```python
from build123d import *

# Parameters (mm, degrees)
F0_W     = 107
F0_H     = 248
F0_W_2   = 99
F0_H_2   = 240
F1_DEPTH = 65
F2_W     = 107
F2_H     = 248
F2_W_2   = 99
F2_H_2   = 240
F3_DEPTH = 4
F4_W     = 58.7
F4_H     = 31.5
F5_DEPTH = 25
F6_R     = 3


with BuildPart() as f1:
    # F0 (on Front) → F1 (new body)
    with BuildSketch(Plane.XZ):
        with Locations((49.5, 120)):
            Rectangle(F0_W, F0_H)
        with Locations((49.5, 120)):
            Rectangle(F0_W_2, F0_H_2, mode=Mode.SUBTRACT)
    extrude(amount=F1_DEPTH)

    # F2 (on face) → F3 (join)
    with BuildSketch(Plane.XZ.offset(65)):
        with Locations((49.5, 120)):
            Rectangle(F2_W, F2_H)
        with Locations((49.5, 120)):
            Rectangle(F2_W_2, F2_H_2, mode=Mode.SUBTRACT)
        with Locations((49.5, 120)):
            Rectangle(F2_W_2, F2_H_2)
    extrude(amount=F3_DEPTH)

    # F4 (on face) → F5 (cut)
    with BuildSketch(Plane.XZ.offset(69)):
        with Locations((49.35, 202.9458682446)):
            Rectangle(F4_W, F4_H)
    extrude(amount=-F5_DEPTH, mode=Mode.SUBTRACT)

    # F6
    f6_edges = [f1.edges().sort_by_distance(p)[0] for p in [
        (-4, -34.5, 244),
        (103, -34.5, 244),
        (-4, -34.5, -4),
        (103, -34.5, -4),
        (49.5, -69, 244),
        (103, -69, 120),
        (-4, -69, 120),
        (49.5, -69, -4),
        (49.35, -69, 218.695868),
        (20, -69, 202.945868),
        (49.35, -69, 187.195868),
        (78.7, -69, 202.945868),
    ]]
    fillet(f6_edges, radius=F6_R)


solid = f1.part
```
Can you work these out from the model? Positions are in its coordinate system, mm. A direction names the side the tool comes from. Coordinates: 2 decimals unless noted, no trailing zeros. Write each loop counter-clockwise with the first axis right and the second up, starting at its lowest first coordinate (ties: lowest second). Pieces come first, ordered by that corner, then holes. Notation, with made-up numbers: M -37.5,3.25 L -13.5,3.25 A28 ccw -13.5,32.25 Z; hole C 39,13.25 d5. An arc over 180 degrees is marked long. Write item = value, one per line. Start each with the question number.
Q1. If I drill on L1, parallel to Z at x = 42.5, y = -39; L2, parallel to X at y = -13, z = 223.5; L3, parallel to Y at x = 93, z = 222, over which ranges is the centre line in solid material (lowest first)? Write a range as [from, to].
Q2. On a 3-axis mill with a long thin cutter (end or side, diameter ignored), from which of +Z, -Z, +X, -X, +Y, -Y can I reach the whole of each face in a straight line? I mean faces 1 (the face through (49, -32, 240)), 2 (the face through (49, -69, 122)). Say none if no direction works.
Q3. Thinking about a two-plate mould opening in X: for faces 3 (the face through (103, -33, 118)), 4 (the face through (49, -65, 122)), 5 (the face through (-2, 0, 121)), 6 (the face through (49, -32, 0)), which applies, released by +X, released by -X, zero draft, split by the parting line, or undercut?
Q4. If we section it at C-C, the plane y = -54: Write out the boundary of the cut face in (x, z).
Q5. If we section it at D-D, the plane z = 146: Write out the boundary of the cut face in (x, y), then the cut area to 3 significant figures.
Q6. If we section it at B-B, the plane x = 72.5: Write out the boundary of the cut face in (y, z), then the cut area to 3 significant figures.
Q7. If we section it at A-A, the plane z = 191: Write out the boundary of the cut face in (x, y), then the cut area to 3 significant figures.
Check sheet entries:
q1.L1 = [-4, 0], [240, 244]
q1.L2 = [-4, 0], [99, 103]
q1.L3 = [-69, -65]
q2.face_1 = +Y
q2.face_2 = +Z, -Z, +X, -X, -Y
q3.face_3 = released by +X
q3.face_4 = undercut
q3.face_5 = zero draft
q3.face_6 = undercut
q4.outline = M -4,-1 A3 ccw -1,-4 L 100,-4 A3 ccw 103,-1 L 103,241 A3 ccw 100,244 L -1,244 A3 ccw -4,241 Z; hole M 0,0 L 99,0 L 99,240 L 0,240 Z
q5.outline = M -4,-66 A3 ccw -1,-69 L 100,-69 A3 ccw 103,-66 L 103,0 L 99,0 L 99,-65 L 0,-65 L 0,0 L -4,0 Z
q5.area = 944 mm²
q6.outline = M -69,-1 A3 ccw -66,-4 L 0,-4 L 0,0 L -65,0 L -65,187.2 L -66,187.2 A3 ccw -69,184.2 Z; M -69,221.7 A3 ccw -66,218.7 L -65,218.7 L -65,240 L 0,240 L 0,244 L -66,244 A3 ccw -69,241 Z
q6.area = 1,380 mm²
q7.outline = M -4,-66 A3 ccw -1,-69 L 17,-69 A3 ccw 20,-66 L 20,-65 L 0,-65 L 0,0 L -4,0 Z; M 78.7,-66 A3 ccw 81.7,-69 L 100,-69 A3 ccw 103,-66 L 103,0 L 99,0 L 99,-65 L 78.7,-65 Z
q7.area = 705 mm²
